```python
from build123d import *

# Parameters (mm, degrees)
SKETCH1_R           = 10
BOSS_EXTRUDE1_DEPTH = 4
SKETCH2_R           = 9
BOSS_EXTRUDE2_DEPTH = 65
SKETCH3_R           = 2
CUT_EXTRUDE1_DEPTH  = 32.5


with BuildPart() as part:
    # Sketch1 → Boss-Extrude1 (new body)
    with BuildSketch(Plane.XY):
        Circle(SKETCH1_R)
    extrude(amount=BOSS_EXTRUDE1_DEPTH)

    # Sketch2 → Boss-Extrude2 (add)
    with BuildSketch(Plane.XY.offset(4)):
        Circle(SKETCH2_R)
    extrude(amount=BOSS_EXTRUDE2_DEPTH)

    # Chamfer4: read off the stored shape, not the designer's step
    # Chamfer4 outline → Chamfer4 (revolve, cut)
    with BuildSketch(Plane.XZ):
        Polygon((9, 69), (7, 69), (9, 67), align=None)
    revolve(axis=Axis((0, 0, 0), (0, 0, 1)), mode=Mode.SUBTRACT)

    # Sketch3 → Cut-Extrude1 (cut, symmetric)
    with BuildSketch(Plane(origin=(0, 0, 0), x_dir=(0, 0, -1), z_dir=(1, 0, 0))):
        with Locations(Location((-62, 0, 0), (0, 0, 180))):
            Circle(SKETCH3_R)
    extrude(amount=CUT_EXTRUDE1_DEPTH, both=True, mode=Mode.SUBTRACT)


solid = part.part
```
Geometry: final body of the model. Coordinates: model frame, mm. A direction names the side the tool comes from. Coordinates: 2 decimals unless noted, no trailing zeros. Order: outer loops, then holes, each group sorted by start corner. A loop starts at its lowest first (then second) coordinate and runs counter-clockwise, first axis right, second up. Notation, with made-up numbers: (29, 10) - (77, 10) arc R27 ccw to (77, 39) - close; hole circle Ø7 at (45.5, -9). An arc over 180 degrees is marked (long way). Write each question's results on one line, items separated by ' | '.
(1) First-contact query: pin 1 Ø4 at (x, z) = (-1.5, 27) entering from -Y; pin 2 Ø12 at (y, z) = (-5, 57) entering from +X; pin 3 Ø2.5 at (y, z) = (0, 62) entering from -X; pin 4 Ø2 at (x, z) = (-7, 12) entering from -Y. Flat tips, straight axial feed; report the tip coordinate or a pass-through.
Values found:
pin 1: stops at y = -9 | pin 2: stops at x = 9 | pin 3: passes through | pin 4: stops at y = -6.71
(2) Line query: line 1 (Z direction, x = -5, y = -0.25); line 2 (X direction, y = 0, z = 48.5). Output: solid intervals per line, ascending. Write a range as [from, to].
Values found:
line 1: z = [0, 60.02], [63.98, 69] | line 2: x = [-9, 9]
(3) Mould query, pull axis Y, two halves, no side actions, for faces 1 (the face through (-2.17, -9.76, 1.97)), 2 (the face through (0, 0, 60)), 3 (the face through (0, 0, 69)). Classes: +Y half, -Y half, draft (parallel to the pull), parting line (faces both ways), or undercut.
Values found:
face 1: parting line | face 2: undercut | face 3: draft
(4) Section query A-A, the plane y = 0. Return the cut outline in (x, z), plus the area to 3 significant figures.
Values found:
outline: (-10, 0) - (10, 0) - (10, 4) - (9, 4) - (9, 60) - (-9, 60) - (-9, 4) - (-10, 4) - close; (-9, 64) - (9, 64) - (9, 67) - (7, 69) - (-7, 69) - (-9, 67) - close | area: 1,170 mm²
(5) Section query C-C, the plane z = 63. Return the cut outline in (x, y).
Values found:
outline: (-8.83, -1.73) arc R9 ccw to (8.83, -1.73) - close; (-8.83, 1.73) - (8.83, 1.73) arc R9 ccw to start
(6) Section query B-B, the plane x = 0. Return the cut outline in (y, z), plus the area to 3 significant figures.
Values found:
outline: (-10, 0) - (10, 0) - (10, 4) - (9, 4) - (9, 67) - (7, 69) - (-7, 69) - (-9, 67) - (-9, 4) - (-10, 4) - close; hole circle Ø4 at (0, 62) | area: 1,230 mm²
(7) Section query D-D, the plane z = 9. Return the cut outline in (x, y), plus the area to 3 significant figures.
Values found:
outline: circle Ø18 at (0, 0) | area: 254 mm²
(8) Set-up query: faces 4 (the face through (0, 0, 0)), 5 (the face through (8.584, 2.703, 35.059)). Return all of +Z, -Z, +X, -X, +Y, -Y with unobstructed straight access to the full face (end or side cutting, diameter ignored); none if empty.
Values found:
face 4: -Z, +X, -X, +Y, -Y | face 5: +Z
